Part model, mm, in its own coordinate system. A direction names the side the tool comes from. Give positions to 0.01 mm unless a question says otherwise; leave off trailing zeros. Loops run counter-clockwise (first coordinate to the right, second up) from the corner with the lowest first, then second, coordinate; pieces in that order, holes last. Notation, with made-up numbers: M -38,-14.75 L 10,-14.75 A8 ccw 10,-6.75 Z; hole C 66,51.5 d5. An arc over 180 degrees is marked long. Answer in a Markdown table with one row per item.
from build123d import *

# Parameters (mm, degrees)
SKETCH1_W           = 60
SKETCH1_H           = 60
BOSS_EXTRUDE1_DEPTH = 3
SKETCH3_R           = 1
CUT_EXTRUDE3_DEPTH  = 43.532340636
SKETCH5_R           = 10.25
CUT_EXTRUDE4_DEPTH  = 43.532340636
SKETCH6_R           = 16
SKETCH6_R_2         = 10.25
BOSS_EXTRUDE2_DEPTH = 1
SKETCH7_R           = 15
SKETCH7_R_2         = 10.25
BOSS_EXTRUDE3_DEPTH = 7


with BuildPart() as part:
    # Sketch1 → Boss-Extrude1 (new body)
    with BuildSketch(Plane(origin=(0, 0, 0), x_dir=(1, 0, 0), z_dir=(0, 1, 0))):
        Rectangle(SKETCH1_W, SKETCH1_H)
    extrude(amount=BOSS_EXTRUDE1_DEPTH)

    # Sketch3 → Cut-Extrude3 (cut, through all)
    with BuildSketch(Plane(origin=(0, 3, 0), x_dir=(1, 0, 0), z_dir=(0, 1, 0))):
        with Locations(Location((-20, 24, 0), (0, 0, 270))):
            Circle(SKETCH3_R)
        with Locations(Location((20, 24, 0), (0, 0, 270))):
            Circle(SKETCH3_R)
        with Locations(Location((-20, -24, 0), (0, 0, 270))):
            Circle(SKETCH3_R)
        with Locations(Location((20, -24, 0), (0, 0, 270))):
            Circle(SKETCH3_R)
    extrude(amount=-CUT_EXTRUDE3_DEPTH, mode=Mode.SUBTRACT)

    # Sketch5 → Cut-Extrude4 (cut, through all)
    with BuildSketch(Plane.XZ):
        with Locations(Location((0, 0, 0), (0, 0, 270))):
            Circle(SKETCH5_R)
    extrude(amount=-CUT_EXTRUDE4_DEPTH, mode=Mode.SUBTRACT)

    # Sketch6 → Boss-Extrude2 (add)
    with BuildSketch(Plane(origin=(0, 3, 0), x_dir=(1, 0, 0), z_dir=(0, 1, 0))):
        with Locations(Location((0, 0, 0), (0, 0, 270))):
            Circle(SKETCH6_R)
        with Locations(Location((0, 0, 0), (0, 0, 90))):
            Circle(SKETCH6_R_2, mode=Mode.SUBTRACT)
    extrude(amount=BOSS_EXTRUDE2_DEPTH)

    # Sketch7 → Boss-Extrude3 (add)
    with BuildSketch(Plane(origin=(0, 3, 0), x_dir=(1, 0, 0), z_dir=(0, 1, 0))):
        with Locations(Location((0, 0, 0), (0, 0, 270))):
            Circle(SKETCH7_R)
        with Locations(Location((0, 0, 0), (0, 0, 90))):
            Circle(SKETCH7_R_2, mode=Mode.SUBTRACT)
    extrude(amount=BOSS_EXTRUDE3_DEPTH)


solid = part.part
(1) Saw through at B-B (z = -24). Write the cut outline in (x, y), plus the area to 3 significant figures.
Recorded:
| item | result |
|---|---|
| outline | M -30,0 L -21,0 L -21,3 L -30,3 Z; M -19,0 L 19,0 L 19,3 L -19,3 Z; M 21,0 L 30,0 L 30,3 L 21,3 Z |
| area | 168 mm^2 |
(2) Saw through at C-C (x = 0). Write the cut outline in (y, z), plus the area to 3 significant figures.
Recorded:
| item | result |
|---|---|
| outline | M 0,-30 L 3,-30 L 3,-16 L 4,-16 L 4,-15 L 10,-15 L 10,-10.25 L 0,-10.25 Z; M 0,10.25 L 10,10.25 L 10,15 L 4,15 L 4,16 L 3,16 L 3,30 L 0,30 Z |
| area | 187 mm^2 |
(3) Saw through at D-D (z = 0). Write the cut outline in (x, y), plus the area to 3 significant figures.
Recorded:
| item | result |
|---|---|
| outline | M -30,0 L -10.25,0 L -10.25,10 L -15,10 L -15,4 L -16,4 L -16,3 L -30,3 Z; M 10.25,0 L 30,0 L 30,3 L 16,3 L 16,4 L 15,4 L 15,10 L 10.25,10 Z |
| area | 187 mm^2 |
(4) Pull direction X, two halves, no side cores. Call faces 1 (the face through (30, 1, 0)), 2 (the face through (-21, 2, -24)), 3 (the face through (19, 2, 24)), 4 (the face through (-14, 0, 0)): +X half, -X half, draft (parallel to the pull), parting line (faces both ways), or undercut.
Recorded:
| item | result |
|---|---|
| face 1 | +X half |
| face 2 | undercut |
| face 3 | undercut |
| face 4 | draft |
(5) Which spindle directions (+Z, -Z, +X, -X, +Y, -Y) get a long thin tool onto all of the face, cutting with end or side? Do faces 5 (the face through (10.006, 4.93, 2.222)), 6 (the face through (-14, 3, -14)). Say none if no direction does.
Recorded:
| item | result |
|---|---|
| face 5 | +Y, -Y |
| face 6 | +Y |
(6) Drill centre lines: line 1 along X through (y, z) = (0.9, 24); line 2 along Z through (x, y) = (0, 7.5). Where is each one in solid material? Low to high.
Recorded:
| item | result |
|---|---|
| line 1 | x = -30 to -21, -19 to 19, 21 to 30 |
| line 2 | z = -15 to -10.25, 10.25 to 15 |
(7) Saw through at A-A (x = -20). Write the cut outline in (y, z), plus the area to 3 significant figures.
Recorded:
| item | result |
|---|---|
| outline | M 0,-30 L 3,-30 L 3,-25 L 0,-25 Z; M 0,-23 L 3,-23 L 3,23 L 0,23 Z; M 0,25 L 3,25 L 3,30 L 0,30 Z |
| area | 168 mm^2 |
(8) Pin check, flat tips, straight feed: pin 1 Ø3 at (x, z) = (20, -24) entering from +Y; pin 2 Ø3 at (x, y) = (1.5, 6.5) entering from -Z; pin 3 Ø5 at (x, y) = (3, 7) entering from +Z. Stop position of each tip, or through.
Recorded:
| item | result |
|---|---|
| pin 1 | stops at y = 3 |
| pin 2 | stops at z = -15 |
| pin 3 | stops at z = 14.99 |
